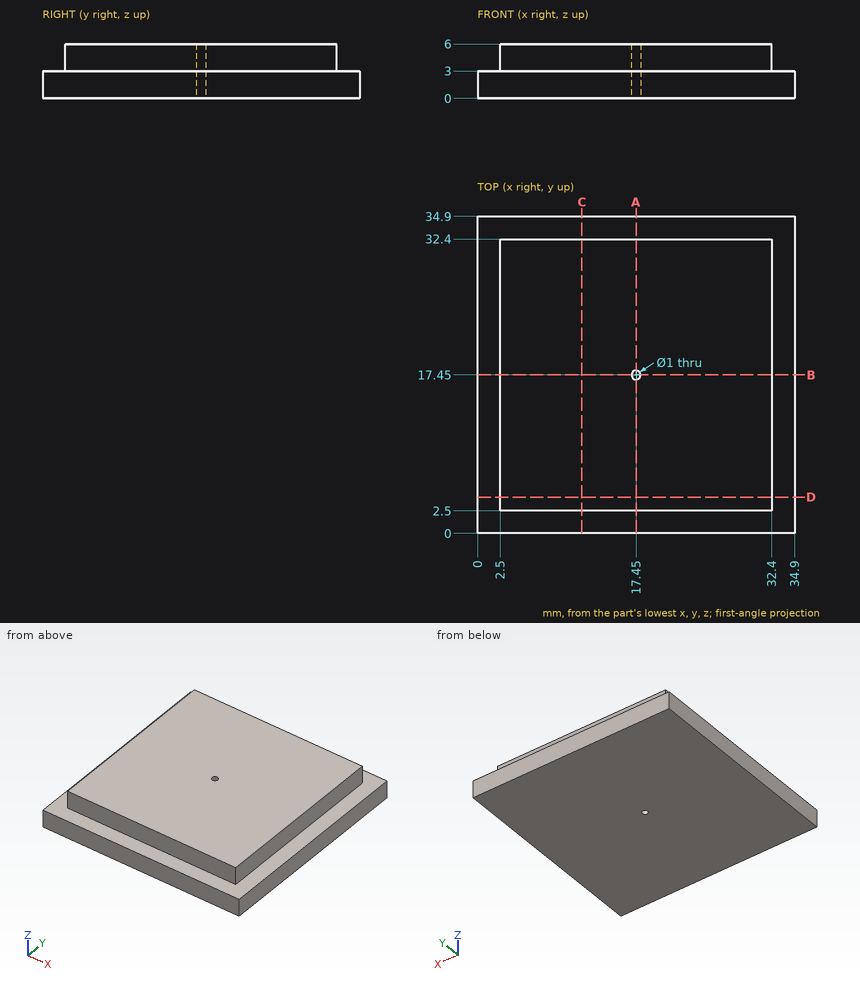
Verification items for this drawing (mm, ordinates from the low corner). Round coordinates to 2 decimals unless told otherwise and drop trailing zeros. Write each loop counter-clockwise with the first axis right and the second up, starting at its lowest first coordinate (ties: lowest second). Pieces come first, ordered by that corner, then holes. Notation, with made-up numbers: (44, 62.5) - (71, 62.5) arc R30 ccw to (71, 101.5) - close; hole circle Ø3 at (13, -0.75). An arc over 180 degrees is marked (long way). Answer as a JSON object with one key per item and string values. Group by question number.
Q1. Thickness scan on line 1 (X direction, y = 9, z = 3.95); line 2 (Y direction, x = 17.45, z = 3.2). Record the ranges inside material, lowest first.
Q2. Section check C-C, the plane x = 11.5. Enter the section's corners in (y, z), plus the area to 3 significant figures.
Q3. Go/stop test with flat-tipped pins: pin 1 Ø2 at (y, z) = (27.5, 4.5) entering from +X; pin 2 Ø1.5 at (y, z) = (4.5, 1) entering from -X; pin 3 Ø1.5 at (x, z) = (14.5, 4.5) entering from +Y. Record where each tip stops, or that it passes through.
Q4. Section check A-A, the plane x = 17.45. Enter the section's corners in (y, z), plus the area to 3 significant figures.
Found:
{
 "1": {"line 1": "x = 2.5 to 32.4", "line 2": "y = 2.5 to 16.95, 17.95 to 32.4"},
 "2": {"outline": "(0, 0) - (34.9, 0) - (34.9, 3) - (32.4, 3) - (32.4, 6) - (2.5, 6) - (2.5, 3) - (0, 3) - close", "area": "194 mm^2"},
 "3": {"pin 1": "stops at x = 32.4", "pin 2": "stops at x = 0", "pin 3": "stops at y = 32.4"},
 "4": {"outline": "(0, 0) - (16.95, 0) - (16.95, 6) - (2.5, 6) - (2.5, 3) - (0, 3) - close; (17.95, 0) - (34.9, 0) - (34.9, 3) - (32.4, 3) - (32.4, 6) - (17.95, 6) - close", "area": "188 mm^2"}
}
